Here's how the part is built. I have some questions about the finished solid (model axes, mm). Face numbers are marked on the shaded views. A direction names the side the tool comes from. Give positions to 0.01 mm unless a question says otherwise; leave off trailing zeros. Loops run counter-clockwise (first coordinate to the right, second up) from the corner with the lowest first, then second, coordinate; pieces in that order, holes last.
Q1. If we section it at A-A (z = 8.5): Please give me the cut outline in (x, y).
Q2. We'd pull the mould along X, two halves only. Please class the marked faces 3, 4 and 5: +X half, -X half, draft (parallel to the pull), parting line (faces both ways), or undercut.
Q3. Will this pin go through, and if not, where does the flat tip stop? P1, Ø5, axis at x = 4, z = 17.5, coming from the +Y side.
Q4. I need wall thicknesses on line 1 (X direction, y = -4.5, z = 26); line 2 (X direction, y = -29.5, z = 4); line 3 (Z direction, x = 23, y = -17). Which ranges of each line are inside material? Lowest first, please.
Q5. If we section it at D-D (z = 13): Please give me the cut outline in (x, y).
Q6. For the marked faces 1 and 2, which set-ups out of +Z, -Z, +X, -X, +Y, -Y let a thin tool reach every point of the face, with its end or its side?
Q7. If we section it at C-C (x = 20): Please give me the cut outline in (y, z).
Q8. If we section it at B-B (y = -13): Please give me the cut outline in (x, z), plus the area to 3 significant figures.
from build123d import *

# Parameters (mm, degrees)
F0_W     = 40
F0_H     = 31.621624
F1_DEPTH = 35
F3_DEPTH = 10
F5_DEPTH = 40


with BuildPart() as f1:
    # F0 (on Top) → F1 (new body)
    with BuildSketch(Plane.XY):
        with Locations((20, -15.810812)):
            Rectangle(F0_W, F0_H)
    extrude(amount=F1_DEPTH)

    # F2 (on face) → F3 (cut)
    with BuildSketch(Plane.XY.offset(35)):
        Polygon((25, -31.621624), (25, -18.624302), (25, 0), (12.5, 0), (12.5, -18.326312), (12.5, -31.621624), align=None)
    extrude(amount=-F3_DEPTH, mode=Mode.SUBTRACT)

    # F4 (on face) → F5 (cut)
    with BuildSketch(Plane.XZ.offset(31.621624)):
        with BuildLine():
            Line((5, 0), (35, 0))
            ThreePointArc((35, 0), (20, 15), (5, 0))
        make_face()
    extrude(amount=-F5_DEPTH, mode=Mode.SUBTRACT)


solid = f1.part
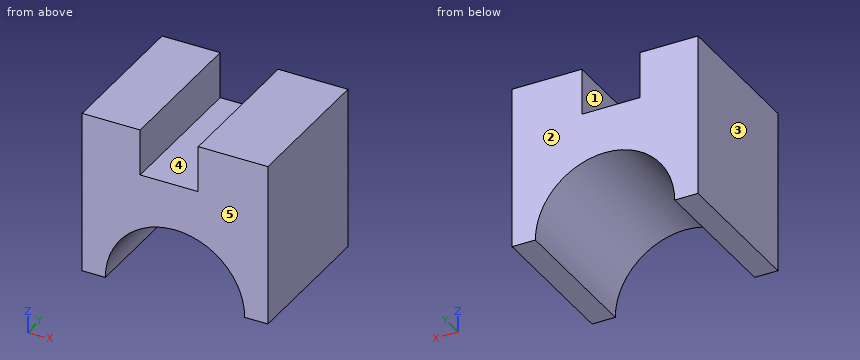
Check sheet entries:
1. outline: (0, -31.62) - (7.64, -31.62) - (7.64, 0) - (0, 0) - close; (32.36, -31.62) - (40, -31.62) - (40, 0) - (32.36, 0) - close
2. face 3: -X half
2. face 4: undercut
2. face 5: draft
3. P1: stops at y = 0
4. line 1: x = 0 to 12.5, 25 to 40
4. line 2: x = 0 to 5.54, 34.46 to 40
4. line 3: z = 14.7 to 25
5. outline: (0, -31.62) - (12.52, -31.62) - (12.52, 0) - (0, 0) - close; (27.48, -31.62) - (40, -31.62) - (40, 0) - (27.48, 0) - close
6. face 1: +Z, +Y, -Y
6. face 2: +Z, -Z, +X, -X, +Y
7. outline: (-31.62, 15) - (0, 15) - (0, 25) - (-31.62, 25) - close
8. outline: (0, 0) - (5, 0) arc R15 cw to (35, 0) - (40, 0) - (40, 35) - (25, 35) - (25, 25) - (12.5, 25) - (12.5, 35) - (0, 35) - close
8. area: 922 mm2
